For this review, take the finished solid that the model builds, in its own axes (mm). A direction names the side the tool comes from. Round coordinates to 2 decimals unless told otherwise and drop trailing zeros. Write each loop counter-clockwise with the first axis right and the second up, starting at its lowest first coordinate (ties: lowest second). Pieces come first, ordered by that corner, then holes. Notation, with made-up numbers: (27, -11.5) - (80, -11.5) arc R17 cw to (80, -4.5) - close; hole circle Ø3 at (-27.5, 25). An arc over 180 degrees is marked (long way). One line per item, written item: value. Start each with the question number.
Q1. For probe 1 along Y at (x, z) = (-2.5, 2.45) (3 decimals); probe 2 along Y at (x, z) = (7.5, 2.75); probe 3 along Y at (x, z) = (5.5, 2) (3 decimals), list the stretches that pass through material, from the lowest coordinate up.
Q2. Add section B-B on y = 31. Write out the cut boundary in (x, z).
Q3. Add section C-C on x = 13.5. Write out the cut boundary in (y, z), and give its area (3 significant figures).
Q4. Add section A-A on y = -47.91. Write out the cut boundary in (x, z), and give its area (3 significant figures).
Q5. Mouldability with a two-part tool opening along X and no side actions: class faces 5 (the face through (-0.52, 27.16, 1.48)), 6 (the face through (5.85, 40, 1)), 7 (the face through (-7, 8.901, 1)) as +X half, -X half, draft (parallel to the pull), parting line (faces both ways), or undercut.
Q6. Clearance check with flat-ended pins moving along their axes: pin 1 Ø1.5 at (y, z) = (44.5, 2) entering from -X; pin 2 Ø1 at (x, z) = (6.5, 1.5) entering from +Y; pin 3 Ø1.6 at (x, z) = (-7, 1) entering from -Y. State where each tip first meets the part, or that it passes through.
Q7. Tool access review of faces 1 (the face through (-5.85, 40, 1)), 2 (the face through (0, -52, 0.49)), 3 (the face through (-5.85, -22, 1)), 4 (the face through (0, 21.951, 1)): name each direction out of +Z, -Z, +X, -X, +Y, -Y from which nothing blocks a thin tool from reaching the whole face with its end or side.
```python
from build123d import *

# Parameters (mm, degrees)
SKETCH1_R           = 2.085
SKETCH1_R_2         = 1.975
SKETCH1_R_3         = 2.4
BOSS_EXTRUDE1_DEPTH = 3
SKETCH2_W           = 2.5
SKETCH2_H           = 2.05
CUT_EXTRUDE1_DEPTH  = 0.49


with BuildPart() as part:
    # Sketch1 → Boss-Extrude1 (new body)
    with BuildSketch(Plane.XY):
        with BuildLine():
            Line((-5.85, 53.045), (-5.85, 27.101350435))
            Line((-5.85, 27.101350435), (-7.9, 27.101350435))
            ThreePointArc((-7.9, 27.101350435), (-17, 18.001350435), (-7.9, 8.901350435))
            Line((-7.9, 8.901350435), (-5.85, 8.901350435))
            Line((-5.85, 8.901350435), (-5.85, -53.045))
            Line((-5.85, -53.045), (-2.685, -53.045))
            Line((-2.685, -53.045), (5.85, -53.045))
            Line((5.85, -53.045), (5.85, 8.901350435))
            Line((5.85, 8.901350435), (7.9, 8.901350435))
            ThreePointArc((7.9, 8.901350435), (17, 18.001350435), (7.9, 27.101350435))
            Line((7.9, 27.101350435), (5.85, 27.101350435))
            Line((5.85, 27.101350435), (5.85, 53.045))
            Line((5.85, 53.045), (-5.85, 53.045))
        make_face()
        with Locations((-2.685, -47.91)):
            Circle(SKETCH1_R, mode=Mode.SUBTRACT)
        with Locations((1.953620485, -44.271379515)):
            Circle(SKETCH1_R_2, mode=Mode.SUBTRACT)
        with BuildLine():
            Line((-7.9, 21.951350435), (7.9, 21.951350435))
            ThreePointArc((7.9, 21.951350435), (11.85, 18.001350435), (7.9, 14.051350435))
            Line((7.9, 14.051350435), (-7.9, 14.051350435))
            ThreePointArc((-7.9, 14.051350435), (-11.85, 18.001350435), (-7.9, 21.951350435))
        make_face(mode=Mode.SUBTRACT)
        with Locations((0, 29.501350435)):
            Circle(SKETCH1_R_3, mode=Mode.SUBTRACT)
    extrude(amount=BOSS_EXTRUDE1_DEPTH)

    # Sketch2 → Cut-Extrude1 (cut)
    with BuildSketch(Plane(origin=(0, 0, 0), x_dir=(-1, 0, 0), z_dir=(0, 0, -1))):
        with Locations((0.045545975, -52.02)):
            Rectangle(SKETCH2_W, SKETCH2_H)
    extrude(amount=-CUT_EXTRUDE1_DEPTH, mode=Mode.SUBTRACT)


solid = part.part
```
Result set:
1. probe 1: y = -53.045 to -49.987, -45.833 to 14.051, 21.951 to 53.045
1. probe 2: y = 8.9 to 14.05, 21.95 to 27.1
1. probe 3: y = -53.045 to 14.051, 21.951 to 53.045
2. outline: (-5.85, 0) - (-1.87, 0) - (-1.87, 3) - (-5.85, 3) - close; (1.87, 0) - (5.85, 0) - (5.85, 3) - (1.87, 3) - close
3. outline: (10.83, 0) - (25.17, 0) - (25.17, 3) - (10.83, 3) - close
3. area: 43.0 mm^2
4. outline: (-5.85, 0) - (-4.77, 0) - (-4.77, 3) - (-5.85, 3) - close; (-0.6, 0) - (5.85, 0) - (5.85, 3) - (-0.6, 3) - close
4. area: 22.6 mm^2
5. face 5: undercut
5. face 6: +X half
5. face 7: draft
6. pin 1: stops at x = -5.85
6. pin 2: stops at y = 27.1
6. pin 3: stops at y = 8.9
7. face 1: +Z, -Z, -X, +Y
7. face 2: -Z, -Y
7. face 3: +Z, -Z, -X, -Y
7. face 4: +Z, -Z
